from build123d import *

# Parameters (mm, degrees)
F3_D           = 3.556
F3_CSINK_D     = 7.112
F3_CSINK_ANGLE = 90
F5_D           = 17.78


with BuildPart() as f1:
    # F0 (on Right) → F1 (revolve)
    with BuildSketch(Plane.YZ):
        with BuildLine():
            ThreePointArc((-2.032, 25.4), (-4.699, 22.57337), (-7.366, 25.4))
            Line((-7.366, 25.4), (-9.398, 25.4))
            Line((-9.398, 25.4), (-9.398, 0))
            Line((-9.398, 0), (0, 0))
            Line((0, 0), (0, 25.4))
            Line((0, 25.4), (-2.032, 25.4))
        make_face()
    revolve(axis=Axis((0, -4.699, 0), (0, 1, 0)))

    # F3 (through all)
    with Locations(Plane(origin=(0, 0, 0), x_dir=(1, 0, 0), z_dir=(0, 1, 0))):
        with Locations((14.2875, 0), (-14.3002, 0)):
            CounterSinkHole(F3_D / 2, F3_CSINK_D / 2, counter_sink_angle=F3_CSINK_ANGLE)

    # F5 (through all)
    with Locations(Plane.XZ.offset(9.398)):
        with Locations((0, 0)):
            Hole(F5_D / 2)


solid = f1.part
Read the model definition and answer for the solid it produces. Units are mm, in the model's axes. Round coordinates to 2 decimals unless told otherwise and drop trailing zeros. Write each loop counter-clockwise with the first axis right and the second up, starting at its lowest first coordinate (ties: lowest second). Pieces come first, ordered by that corner, then holes. Notation, with made-up numbers: (88.25, -25.75) - (106.25, -25.75) arc R19 ccw to (106.25, -15.75) - close; hole circle Ø11 at (-4, -4.75). An arc over 180 degrees is marked (long way). One line per question, with ' | ' between items. Start each with the question number.
1. For a pull along Z with two mould halves and no side action, classify faces 1 (the face through (-24.796, -1.03, -5.506)), 2 (the face through (1.93, -4.63, -8.68)), 3 (the face through (0, -9.398, 11)) as +Z half, -Z half, draft (parallel to the pull), parting line (faces both ways), or undercut.
2. Section A-A (z = 0) is taken. Determine the outline of the cut face in (x, y).
3. Find the intervals of material crossed by probe 1 along Z at (x, y) = (1, -2.75); probe 2 along Z at (x, y) = (14, -8.5); probe 3 along X at (y, z) = (-0.75, -5.5), in increasing order. Write a range as [from, to].
4. Section B-B (y = -3.5) is taken. Determine the outline of the cut face in (x, z), and give its area (3 significant figures).
5. Each of these flat-tipped pins is pushed along its axis until it touches: pin 1 (4 mm diameter, centred on x = -14.3, z = 0, fed in from +Y); pin 2 (5 mm diameter, centred on y = -1, z = 4.5, fed in from -X); pin 3 (1 mm diameter, centred on x = -12.5, y = -2, fed in from +Z). Where does it stop, or does it pass through?
Filled in:
1) face 1: parting line | face 2: undercut | face 3: draft
2) outline: (-25.4, -9.4) - (-16.08, -9.4) - (-16.08, -1.78) - (-17.86, 0) - (-25.4, 0) - (-25.4, -2.03) arc R2.67 cw (long way) to (-25.4, -7.37) - close; (-12.52, -9.4) - (-8.89, -9.4) - (-8.89, 0) - (-10.74, 0) - (-12.52, -1.78) - close; (8.89, -9.4) - (12.51, -9.4) - (12.51, -1.78) - (10.73, 0) - (8.89, 0) - close; (16.07, -9.4) - (25.4, -9.4) - (25.4, -7.37) arc R2.67 cw (long way) to (25.4, -2.03) - (25.4, 0) - (17.84, 0) - (16.07, -1.78) - close
3) probe 1: [-23.4, -8.83], [8.83, 23.4] | probe 2: [-21.19, -1.75], [1.75, 21.19] | probe 3: [-24.8, -6.98], [6.98, 24.8]
4) outline: circle Ø45.72 at (0, 0); hole circle Ø3.56 at (-14.3, 0); hole circle Ø17.78 at (0, 0); hole circle Ø3.56 at (14.29, 0) | area: 1,370 mm²
5) pin 1: y = -1.56 | pin 2: x = -25.32 | pin 3: z = 22.39
